Could you check a few things on this drawing? It's one solid part, dimensions in mm from its lowest x, y, z. A direction names the side the tool comes from. Give positions to 0.01 mm unless a question says otherwise; leave off trailing zeros. Order: outer loops, then holes, each group sorted by start corner. A loop starts at its lowest first (then second) coordinate and runs counter-clockwise, first axis right, second up.
Item 1: If we mould it in two halves opening along Y, with no side actions, what happens to the marked faces 4, 5, 6 and 7? For each: +Y half, -Y half, draft (parallel to the pull), parting line (faces both ways), or undercut.
Item 2: I want a section at C-C, the plane z = 34. Write out the boundary of the cut face in (x, y).
Item 3: I want a section at D-D, the plane y = 508.5. Write out the boundary of the cut face in (x, z), then the cut area to 3 significant figures.
Item 4: I want a section at A-A, the plane z = 102. Write out the boundary of the cut face in (x, y), then the cut area to 3 significant figures.
Item 5: If I drill on line 1 along Z through (x, y) = (44, 526.5); line 2 along Y through (x, z) = (53, 77); line 3 along Y through (x, z) = (9.5, 121.5), over which ranges is the centre line in solid material (lowest first)?
Item 6: Which directions (+Z, -Z, +X, -X, +Y, -Y) give clear straight access to the entire face, cutting with the end or side of a thin tool? Please do the marked faces 1, 2 and 3.
Item 7: I'm going to push flat-ended pins straight in: pin 1 Ø1 at (x, y) = (46.5, 374) entering from -Z; pin 2 Ø10 at (y, z) = (379.5, 99) entering from +X; pin 3 Ø4 at (x, z) = (37.5, 32.5) entering from -Y (1 decimal). Where does each tip first touch, or does it pass through?
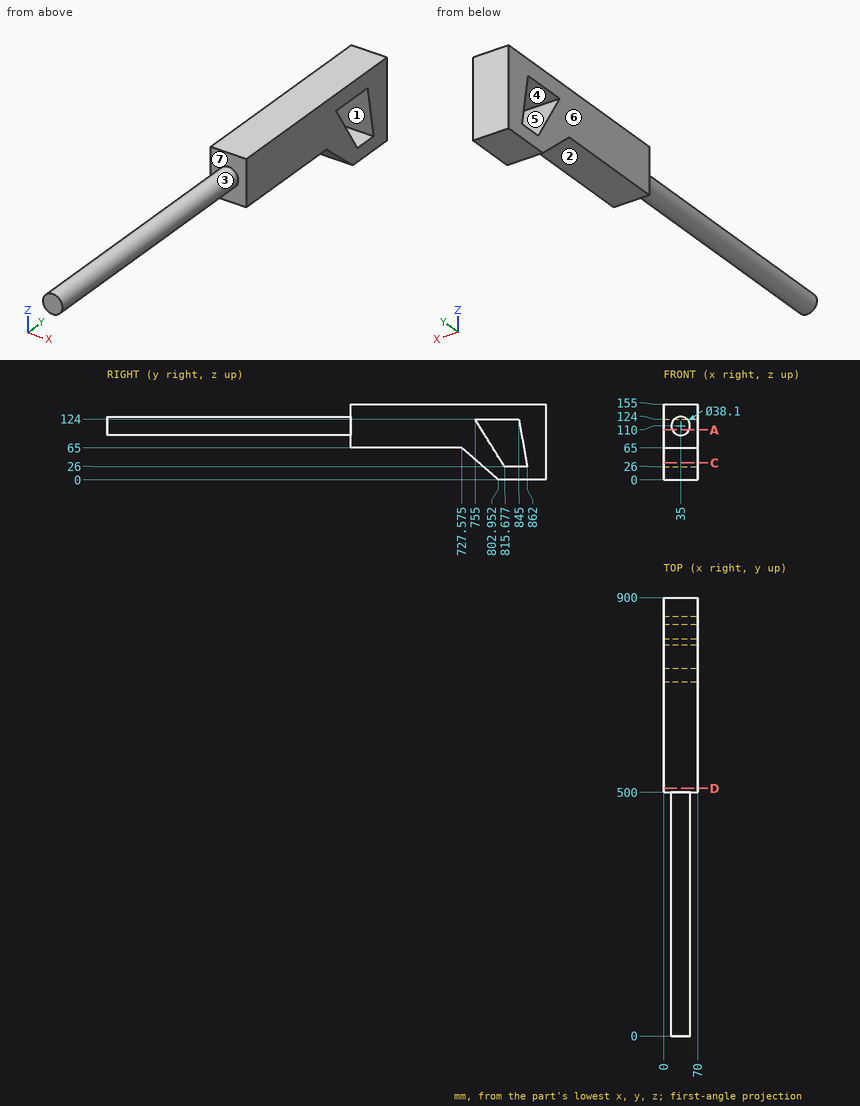
Results list:
1. face 4: undercut
1. face 5: undercut
1. face 6: draft
1. face 7: -Y half
2. outline: (0, 763.52) - (70, 763.52) - (70, 810.72) - (0, 810.72) - close; (0, 860.61) - (70, 860.61) - (70, 900) - (0, 900) - close
3. outline: (0, 65) - (70, 65) - (70, 155) - (0, 155) - close
3. area: 6,300 mm2
4. outline: (0, 500) - (17.71, 500) - (17.71, 0) - (52.29, 0) - (52.29, 500) - (70, 500) - (70, 768.62) - (0, 768.62) - close; (0, 848.82) - (70, 848.82) - (70, 900) - (0, 900) - close
4. area: 39,700 mm2
5. line 1: z = 65 to 155
5. line 2: y = 500 to 784.1, 853.15 to 900
5. line 3: y = 500 to 756.55, 845.43 to 900
6. face 1: +X, -X
6. face 2: -Z, +X, -X, -Y
6. face 3: -Y
7. pin 1: stops at z = 94.45
7. pin 2: stops at x = 53.08
7. pin 3: stops at y = 762.9
